from build123d import *

# Parameters (mm, degrees)
BOSS_EXTRUDE1_DEPTH                            = 3
CSK_FOR_M3_FLAT_HEAD_MACHINE_SCREW1_AT_2_COUNT = 2
CSK_FOR_M3_FLAT_HEAD_MACHINE_SCREW1_AT_2_PITCH = 15.85
CSK_FOR_M3_FLAT_HEAD_MACHINE_SCREW1_AT_3_COUNT = 2
CSK_FOR_M3_FLAT_HEAD_MACHINE_SCREW1_AT_3_PITCH = 27.4530053
CSK_FOR_M3_FLAT_HEAD_MACHINE_SCREW1_AT_4_COUNT = 2
CSK_FOR_M3_FLAT_HEAD_MACHINE_SCREW1_AT_4_PITCH = 31.7
CSK_FOR_M3_FLAT_HEAD_MACHINE_SCREW1_AT_5_COUNT = 2
CSK_FOR_M3_FLAT_HEAD_MACHINE_SCREW1_AT_5_PITCH = 27.4530053
CSK_FOR_M3_FLAT_HEAD_MACHINE_SCREW1_AT_6_COUNT = 2
CSK_FOR_M3_FLAT_HEAD_MACHINE_SCREW1_AT_6_PITCH = 15.85
SKETCH6_W                                      = 40
SKETCH6_H                                      = 3
BOSS_EXTRUDE2_DEPTH                            = 41
SKETCH7_R                                      = 1.7
CUT_EXTRUDE1_DEPTH                             = 3
FILLET1_R                                      = 3
FILLET2_R                                      = 5


with BuildPart() as part:
    # Sketch2 → Boss-Extrude1 (new body)
    with BuildSketch(Plane.XY):
        with BuildLine():
            Line((0, 0), (40, 0))
            Line((40, 0), (40, 25.75))
            ThreePointArc((40, 25.75), (20, 45.75), (0, 25.75))
            Line((0, 25.75), (0, 0))
        make_face()
        with BuildLine():
            Line((26.240819183, 17.25), (26.240819183, 31.15))
            ThreePointArc((26.240819183, 31.15), (19.790819183, 37.6), (13.340819183, 31.15))
            Line((13.340819183, 31.15), (13.340819183, 17.25))
            ThreePointArc((13.340819183, 17.25), (19.790819183, 10.8), (26.240819183, 17.25))
        make_face(mode=Mode.SUBTRACT)
    extrude(amount=-BOSS_EXTRUDE1_DEPTH)

    # Sketch4 → CSK for M3 Flat Head Machine Screw1 (revolve, cut)
    with BuildSketch(Plane(origin=(4.15, 25.75, 0), x_dir=(0, -1, 0), z_dir=(1, 0, 0))):
        Polygon((0, 0), (0, 3), (1.7, 3), (1.7, 1.45), (3.15, 0), align=None)
    csk_for_m3_flat_head_machine_screw1 = revolve(axis=Axis((4.15, 25.75, 6.35), (0, 0, -1)), mode=Mode.SUBTRACT)

    # CSK for M3 Flat Head Machine Screw1 at 2: CSK for M3 Flat Head Machine Screw1 ×2
    with Locations(*[Vector(0.49999999999999317, 0.8660254037844426, 0) * (i * CSK_FOR_M3_FLAT_HEAD_MACHINE_SCREW1_AT_2_PITCH) for i in range(1, CSK_FOR_M3_FLAT_HEAD_MACHINE_SCREW1_AT_2_COUNT)]):
        add(csk_for_m3_flat_head_machine_screw1, mode=Mode.SUBTRACT)

    # CSK for M3 Flat Head Machine Screw1 at 3: CSK for M3 Flat Head Machine Screw1 ×2
    with Locations(*[Vector(0.8660254037844348, 0.5000000000000067, 0) * (i * CSK_FOR_M3_FLAT_HEAD_MACHINE_SCREW1_AT_3_PITCH) for i in range(1, CSK_FOR_M3_FLAT_HEAD_MACHINE_SCREW1_AT_3_COUNT)]):
        add(csk_for_m3_flat_head_machine_screw1, mode=Mode.SUBTRACT)

    # CSK for M3 Flat Head Machine Screw1 at 4: CSK for M3 Flat Head Machine Screw1 ×2
    with Locations(*[(i * CSK_FOR_M3_FLAT_HEAD_MACHINE_SCREW1_AT_4_PITCH, 0, 0) for i in range(1, CSK_FOR_M3_FLAT_HEAD_MACHINE_SCREW1_AT_4_COUNT)]):
        add(csk_for_m3_flat_head_machine_screw1, mode=Mode.SUBTRACT)

    # CSK for M3 Flat Head Machine Screw1 at 5: CSK for M3 Flat Head Machine Screw1 ×2
    with Locations(*[Vector(0.8660254037844427, -0.49999999999999306, 0) * (i * CSK_FOR_M3_FLAT_HEAD_MACHINE_SCREW1_AT_5_PITCH) for i in range(1, CSK_FOR_M3_FLAT_HEAD_MACHINE_SCREW1_AT_5_COUNT)]):
        add(csk_for_m3_flat_head_machine_screw1, mode=Mode.SUBTRACT)

    # CSK for M3 Flat Head Machine Screw1 at 6: CSK for M3 Flat Head Machine Screw1 ×2
    with Locations(*[Vector(0.5000000000000067, -0.8660254037844349, 0) * (i * CSK_FOR_M3_FLAT_HEAD_MACHINE_SCREW1_AT_6_PITCH) for i in range(1, CSK_FOR_M3_FLAT_HEAD_MACHINE_SCREW1_AT_6_COUNT)]):
        add(csk_for_m3_flat_head_machine_screw1, mode=Mode.SUBTRACT)

    # Sketch6 → Boss-Extrude2 (add)
    with BuildSketch(Plane(origin=(0, 0, -3), x_dir=(-1, 0, 0), z_dir=(0, 0, -1))):
        with Locations((-20, 1.5)):
            Rectangle(SKETCH6_W, SKETCH6_H)
    extrude(amount=BOSS_EXTRUDE2_DEPTH)

    # Sketch7 → Cut-Extrude1 (cut)
    with BuildSketch(Plane.XZ):
        with Locations(Location((5, -37.5, 0), (0, 0, 270))):
            Circle(SKETCH7_R)
        with Locations(Location((5, -13.5, 0), (0, 0, 270))):
            Circle(SKETCH7_R)
        with Locations(Location((35, -37.5, 0), (0, 0, 270))):
            Circle(SKETCH7_R)
        with Locations(Location((35, -13.5, 0), (0, 0, 270))):
            Circle(SKETCH7_R)
    extrude(amount=-CUT_EXTRUDE1_DEPTH, mode=Mode.SUBTRACT)

    # Fillet1
    fillet1_edges = [part.edges().sort_by_distance(p)[0] for p in [
        (0, 1.5, -44),
        (40, 1.5, -44),
    ]]
    fillet(fillet1_edges, radius=FILLET1_R)

    # Fillet2
    fillet2_edges = [part.edges().sort_by_distance(p)[0] for p in [
        (20, 0, 0),
    ]]
    fillet(fillet2_edges, radius=FILLET2_R)


solid = part.part
Can you work these out from the model? Positions are in its coordinate system, mm. A direction names the side the tool comes from. Round coordinates to 2 decimals unless told otherwise and drop trailing zeros. Write each loop counter-clockwise with the first axis right and the second up, starting at its lowest first coordinate (ties: lowest second). Pieces come first, ordered by that corner, then holes. Notation, with made-up numbers: M 56.5,81 L 85.5,81 A34 cw 85.5,112 Z; hole C 85.25,-4.5 d8. An arc over 180 degrees is marked long. Use a Markdown table: item, result.
Item 1: For pin 1 Ø12 at (x, z) = (21, -13.5) entering from +Y; pin 2 Ø4.5 at (x, y) = (27.93, 39.48) entering from +Z; pin 3 Ø6 at (x, y) = (25, 30.5) entering from +Z; pin 4 Ø5.5 at (x, y) = (4.15, 25.75) entering from -Z, each with a flat end and sliding along its axis, tell me the tip position at first contact or that it passes through.
Found:
| item | result |
|---|---|
| pin 1 | stops at y = 3 |
| pin 2 | stops at z = -0.89 |
| pin 3 | stops at z = 0 |
| pin 4 | stops at z = -3 |
Item 2: If I drill on line 1 along X through (y, z) = (25.75, -1.8); line 2 along Y through (x, z) = (6, -39); line 3 along Y through (x, z) = (13, -1.5) (3 decimals), over which ranges is the centre line in solid material (lowest first)? Write a range as [from, to].
Found:
| item | result |
|---|---|
| line 1 | x = [0, 2.45], [5.85, 13.34], [26.24, 34.15], [37.55, 40] |
| line 2 | y = [0, 3] |
| line 3 | y = [1.429, 10.597], [13.45, 38.05], [40.903, 44.485] |
Item 3: I want a section at C-C (x = 17). List the corners of the cut face in (y, z) for me, and give its area (3 significant figures).
Found:
| item | result |
|---|---|
| outline | M 0,-44 L 3,-44 L 3,-3 L 11.44,-3 L 11.44,0 L 5,0 A5 ccw 0,-5 Z; M 36.96,-3 L 45.52,-3 L 45.52,0 L 36.96,0 Z |
| area | 178 mm2 |
Item 4: I want a section at A-A (z = -37.5). List the corners of the cut face in (x, y) for me, and give its area (3 significant figures).
Found:
| item | result |
|---|---|
| outline | M 0,0 L 3.3,0 L 3.3,3 L 0,3 Z; M 6.7,0 L 33.3,0 L 33.3,3 L 6.7,3 Z; M 36.7,0 L 40,0 L 40,3 L 36.7,3 Z |
| area | 99.6 mm2 |
Item 5: We'd pull the mould along X, two halves only. Please class faces 3 (the face through (11.564, 10.402, -2.214)), 4 (the face through (0.9, 1.52, -43.14)), 5 (the face through (29, 20, -3)): released by +X, released by -X, zero draft, split by the parting line, or undercut.
Found:
| item | result |
|---|---|
| face 3 | undercut |
| face 4 | released by -X |
| face 5 | zero draft |
Item 6: I want a section at B-B (x = 35.85). List the corners of the cut face in (y, z) for me.
Found:
| item | result |
|---|---|
| outline | M 0,-44 L 3,-44 L 3,-38.97 L 0,-38.97 Z; M 0,-36.03 L 3,-36.03 L 3,-14.97 L 0,-14.97 Z; M 0,-12.03 L 3,-12.03 L 3,-3 L 24.05,-3 L 24.05,-1.45 L 22.6,0 L 5,0 A5 ccw 0,-5 Z; M 27.45,-3 L 37.95,-3 L 37.95,0 L 28.9,0 L 27.45,-1.45 Z |
Item 7: I want a section at D-D (x = 5). State how many separate pieces and enclosed holes the cut face has, and give its area (3 significant figures).
Found:
| item | result |
|---|---|
| separate pieces | 4 |
| enclosed holes | 0 |
| area | 203 mm2 |
Item 8: Which directions (+Z, -Z, +X, -X, +Y, -Y) give clear straight access to the entire face, cutting with the end or side of a thin tool? Please do faces 1 (the face through (13.341, 24, -1)), 2 (the face through (3.97, 1.48, -36.15)).
Found:
| item | result |
|---|---|
| face 1 | +Z, -Z |
| face 2 | +Y, -Y |
